```python
from build123d import *

# Parameters (mm, degrees)
SKETCH2_R                  = 10.65
BOSS_EXTRUDE1_DEPTH        = 1.4
M2_CLEARANCE_HOLE1_D       = 2.362
M2_CLEARANCE_HOLE1_DEPTH   = 5
M2_CLEARANCE_HOLE2_D       = 2.362
M2_CLEARANCE_HOLE2_DEPTH   = 9
M3_5_CLEARANCE_HOLE1_D     = 3.83
M3_5_CLEARANCE_HOLE1_DEPTH = 5
M2_CLEARANCE_HOLE3_D       = 2.362
M2_CLEARANCE_HOLE3_DEPTH   = 5
CHAMFER1_SIZE              = 0.498


with BuildPart() as part:
    # Sketch1 → Revolve1 (revolve)
    with BuildSketch(Plane(origin=(0, 0, 0), x_dir=(-1, 0, 0), z_dir=(0, 0, -1))):
        with BuildLine():
            Line((-2.413, -4), (0, -4))
            Line((0, -4), (0, 24))
            Line((0, 24), (-11.5, 24))
            Line((-11.5, 24), (-11.5, 0))
            Line((-11.5, 0), (-8.835106781, 0))
            ThreePointArc((-8.835106781, 0), (-8.128, -0.5), (-7.420893219, 0))
            Line((-7.420893219, 0), (-3.602106781, 0))
            ThreePointArc((-3.602106781, 0), (-3.092512244, -0.473525337), (-2.413, -0.324609433))
            Line((-2.413, -0.324609433), (-2.413, -4))
        make_face()
    revolve(axis=Axis((0, -4, 0), (0, 1, 0)))

    # Sketch2 → Boss-Extrude1 (add)
    with BuildSketch(Plane(origin=(0, 24, 0), x_dir=(-1, 0, 0), z_dir=(0, 1, 0))):
        Circle(SKETCH2_R)
    extrude(amount=BOSS_EXTRUDE1_DEPTH)

    # M2 Clearance Hole1
    with Locations(Plane(origin=(0, 0, 0), x_dir=(-1, 0, 0), z_dir=(0, -1, 0))):
        with Locations((-5.5, 0), (5.5, 0)):
            Hole(M2_CLEARANCE_HOLE1_D / 2, depth=M2_CLEARANCE_HOLE1_DEPTH)

    # M2 Clearance Hole2
    with Locations(Plane(origin=(0, -4, 0), x_dir=(-1, 0, 0), z_dir=(0, -1, 0))):
        with Locations((0, 0)):
            Hole(M2_CLEARANCE_HOLE2_D / 2, depth=M2_CLEARANCE_HOLE2_DEPTH)

    # M3.5 Clearance Hole1
    with Locations(Plane(origin=(0, 25.4, 0), x_dir=(1, 0, 0), z_dir=(0, 1, 0))):
        with Locations((0, 0)):
            Hole(M3_5_CLEARANCE_HOLE1_D / 2, depth=M3_5_CLEARANCE_HOLE1_DEPTH)

    # M2 Clearance Hole3
    with Locations(Plane(origin=(0, 25.4, 0), x_dir=(1, 0, 0), z_dir=(0, 1, 0))):
        with Locations((5.5, 0), (-5.5, 0)):
            Hole(M2_CLEARANCE_HOLE3_D / 2, depth=M2_CLEARANCE_HOLE3_DEPTH)

    # Chamfer1
    chamfer1_edges = [part.edges().sort_by_distance(p)[0] for p in [
        (-2.413, -4, 0),
        (1.915, 25.4, 0),
        (-11.5, 0, 0),
    ]]
    chamfer(chamfer1_edges, length=CHAMFER1_SIZE)


solid = part.part
```
The listing builds one solid part. Answer for the finished solid, in the listing's coordinates (mm). A direction names the side the tool comes from. Round coordinates to 2 decimals unless told otherwise and drop trailing zeros. Loops run counter-clockwise (first coordinate to the right, second up) from the corner with the lowest first, then second, coordinate; pieces in that order, holes last.
1) Consider line 1 (Z direction, x = 0, y = 1); line 2 (Z direction, x = 0, y = 21.5) (3 decimals); line 3 (Y direction, x = -8.5, z = 6). Determine where each line is inside the solid, lowest interval first.
Outcome:
line 1: z = -11.5 to -1.18, 1.18 to 11.5
line 2: z = -11.5 to -1.915, 1.915 to 11.5
line 3: y = 0 to 25.4
2) A cutting plane is placed at D-D on y = 22. Determine the outline of the cut face in (x, z) (3 decimals).
Outcome:
outline: circle Ø23 at (0, 0); hole circle Ø2.362 at (-5.5, 0); hole circle Ø3.83 at (0, 0); hole circle Ø2.362 at (5.5, 0)
3) For faces 4 (the face through (3, 25.4, 0)), 5 (the face through (-6, 5, 0)), 6 (the face through (-6.63, 22.86, -0.35)), determine the directions among +Z, -Z, +X, -X, +Y, -Y from which every point of the face is accessible in a straight line to the end or side of a thin tool.
Outcome:
face 4: +Z, -Z, +X, -X, +Y
face 5: -Y
face 6: +Y
4) A cutting plane is placed at C-C on y = 4. Determine the outline of the cut face in (x, z), plus the area to 3 significant figures.
Outcome:
outline: circle Ø23 at (0, 0); hole circle Ø2.36 at (-5.5, 0); hole circle Ø2.36 at (0, 0); hole circle Ø2.36 at (5.5, 0)
area: 402 mm2
5) Given P1, Ø1.9, axis at x = 0, z = 0, coming from the -Y side; P2, Ø1.9, axis at x = 0.5, z = -1, coming from the +Y side; P3, Ø2.5, axis at x = 6, z = 0.5, coming from the +Y side; P4, Ø4, axis at x = -5.5, z = 0, coming from the -Y side, each flat-ended and moving along its own axis, determine where each tip first touches the part or whether it passes through.
Outcome:
P1: stops at y = 5
P2: stops at y = 25.06
P3: stops at y = 25.4
P4: stops at y = -0.19
6) A cutting plane is placed at B-B on y = 12.25. Determine the outline of the cut face in (x, z).
Outcome:
outline: circle Ø23 at (0, 0)
7) For a pull along X with two mould halves and no side action, classify faces 1 (the face through (-8, 24, 8)), 2 (the face through (6, 20.4, 0)), 3 (the face through (-10.158, 24.69, 3.199)) as released by +X, released by -X, zero draft, split by the parting line, or undercut.
Outcome:
face 1: zero draft
face 2: undercut
face 3: split by the parting line
